```python
from build123d import *

# Parameters (mm, degrees)
F0_R      = 15.5
F1_DEPTH  = 40
F4_DEPTH  = 40
F5_R      = 1
F6_R      = 14.25
F7_DEPTH  = 34
F8_SIZE   = 2
F10_DEPTH = 20
F13_R     = 4


with BuildPart() as f1:
    # F0 (on Top) → F1 (new body)
    with BuildSketch(Plane.XY):
        Circle(F0_R)
    extrude(amount=F1_DEPTH)

    # F3 (on offset) → F4 (cut)
    with BuildSketch(Plane.XZ.offset(20)):
        with BuildLine():
            Line((19.5, 11.75), (19.5, 17.75))
            Line((19.5, 17.75), (3.5, 17.75))
            Line((3.5, 17.75), (3.5, 23.5))
            ThreePointArc((3.5, 23.5), (0, 27), (-3.5, 23.5))
            Line((-3.5, 23.5), (-3.5, 6))
            ThreePointArc((-3.5, 6), (0, 2.5), (3.5, 6))
            Line((3.5, 6), (3.5, 11.75))
            Line((3.5, 11.75), (19.5, 11.75))
        make_face()
    extrude(amount=-F4_DEPTH, mode=Mode.SUBTRACT)

    # F5
    f5_edges = [f1.edges().sort_by_distance(p)[0] for p in [
        (0, -15.5, 27),
        (0, 15.5, 27),
        (12.134661, -9.643651, 17.75),
        (12.134661, 9.643651, 17.75),
        (12.134661, -9.643651, 11.75),
        (12.134661, 9.643651, 11.75),
        (-3.5, -15.099669, 14.75),
        (-3.5, 15.099669, 14.75),
        (3.5, 0, 17.75),
        (3.5, 0, 11.75),
    ]]
    fillet(f5_edges, radius=F5_R)

    # F6 (on face) → F7 (join)
    with BuildSketch(Plane(origin=(0, 0, 0), x_dir=(1, 0, 0), z_dir=(0, 0, -1))):
        Circle(F6_R)
    extrude(amount=F7_DEPTH)

    # F8
    f8_edges = [f1.edges().sort_by_distance(p)[0] for p in [
        (-14.25, 0, -34),
    ]]
    chamfer(f8_edges, length=F8_SIZE)

    # F9 (on face) → F10 (cut)
    with BuildSketch(Plane(origin=(0, 0, -34), x_dir=(1, 0, 0), z_dir=(0, 0, -1))):
        Polygon((3, 21.450706), (3, 3), (33.327906, 3), align=None)
        Polygon((-23, 3), (-3, 3), (-3, 21.450706), align=None)
        Polygon((-3, -23), (-3, -3), (-23, -3), align=None)
        Polygon((33.327906, -3), (3, -3), (3, -23), align=None)
    extrude(amount=-F10_DEPTH, mode=Mode.SUBTRACT)

    # F11 (on Front) → F12 (revolve, cut)
    with BuildSketch(Plane.XZ):
        with BuildLine():
            ThreePointArc((0.1, 40), (14.242136, 34.142136), (20.1, 20))
            Line((20.1, 20), (20.1, 40))
            Line((20.1, 40), (0.1, 40))
        make_face()
    revolve(axis=Axis((0, 0, 20), (0, 0, 1)), mode=Mode.SUBTRACT)

    # F13
    f13_edges = [f1.edges().sort_by_distance(p)[0] for p in [
        (-15.5, 0, 32.760878),
    ]]
    fillet(f13_edges, radius=F13_R)


solid = f1.part
```
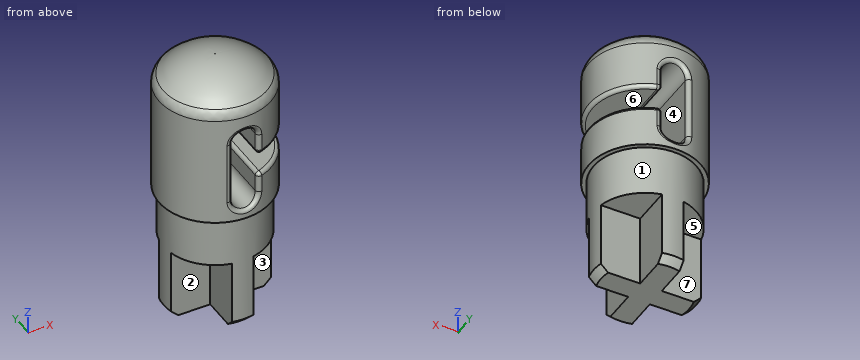
For this review, take the finished solid that the model builds, in its own axes (mm). Face numbers are marked on the shaded views. A direction names the side the tool comes from. Round coordinates to 2 decimals unless told otherwise and drop trailing zeros. Write each loop counter-clockwise with the first axis right and the second up, starting at its lowest first coordinate (ties: lowest second). Pieces come first, ordered by that corner, then holes. Notation, with made-up numbers: (48.5, 20) -> (54.5, 20) arc R33 ccw to (54.5, 51) -> close; hole circle Ø6 at (75, 34). An arc over 180 degrees is marked (long way). One line per question, with ' | ' between items. Start each with the question number.
(1) For line 1 along X through (y, z) = (9.5, 19); line 2 along X through (y, z) = (-3.5, -16.5), list the stretches that pass through material, from the lowest coordinate up. Write a range as from..to.
(2) Add section B-B, the plane z = 13. Write out the cut boundary in (x, y).
(3) Mouldability with a two-part tool opening along Z and no side actions: class the marked faces 5, 6 and 7 as released by +Z, released by -Z, zero draft, split by the parting line, or undercut.
(4) Add section C-C, the plane z = -2.5. Write out the cut boundary in (x, y).
(5) Tool access review of the marked faces 1, 2, 3 and 4: name each direction out of +Z, -Z, +X, -X, +Y, -Y from which nothing blocks a thin tool from reaching the whole face with its end or side.
(6) Insertion check: P1, Ø1.4, axis at y = 6.5, z = 8.5, coming from the -X side; P2, Ø4, axis at y = 10, z = -9, coming from the -X side; P3, Ø1.5, axis at x = -9, y = -8.5, coming from the -Z side. Each pin has a flat end and moves straight along its axis. Give the tip position at first contact, or say it passes through.
(7) Add section A-A, the plane z = -20. Write out the cut boundary in (x, y).
Answer list:
1) line 1: -12.25..-3.5, 3.5..12.25 | line 2: -3..3
2) outline: (-4.81, -14.73) arc R1 ccw to (-3.5, -13.78) -> (-3.5, 13.78) arc R1 ccw to (-4.81, 14.73) arc R15.5 ccw to start
3) face 5: released by -Z | face 6: undercut | face 7: zero draft
4) outline: circle Ø28.5 at (0, 0)
5) face 1: -Z | face 2: -Z, -X, -Y | face 3: -Z, +X, -Y | face 4: +Y, -Y
6) P1: x = -14.37 | P2: x = -11.79 | P3: z = -14
7) outline: (-13.93, -3) -> (-3, -3) -> (-3, -13.93) arc R14.25 ccw to (3, -13.93) -> (3, -3) -> (13.93, -3) arc R14.25 ccw to (13.93, 3) -> (3, 3) -> (3, 13.93) arc R14.25 ccw to (-3, 13.93) -> (-3, 3) -> (-13.93, 3) arc R14.25 ccw to start
